from build123d import *

# Parameters (mm, degrees)
BASE_R                       = 9.5
BODY_DEPTH                   = 4.5
BASE_2_R                     = 4.53
SPLINE_EXTRUSION_BACK_DEPTH  = 1.34
BASE_3_R                     = 4.02
BASE_3_R_2                   = 3.27
SPLINE_EXTRUSION_FRONT_DEPTH = 0.6
FRONT_START                  = -0.9
FRONT_BASE_R                 = 3.27
FRONT_RECESSION_DEPTH        = 0.9
SPLINE_DEPTH                 = 4.3
CENTER_SCREW_HOLE_DEPTH      = 0.64
SCREW_HOLE_SKETCH_R          = 1
SCREW_HOLES_DEPTH            = 15.649423197


with BuildPart() as part:
    # base → body (new body)
    with BuildSketch(Plane.XY):
        Circle(BASE_R)
    extrude(amount=BODY_DEPTH)

    # base 2 → spline extrusion back (add)
    with BuildSketch(Plane(origin=(0, 0, 0), x_dir=(-1, 0, 0), z_dir=(0, 0, -1))):
        with Locations(Location((0, 0, 0), (0, 0, 180))):
            Circle(BASE_2_R)
    extrude(amount=SPLINE_EXTRUSION_BACK_DEPTH)

    # base 3 → spline extrusion front (add)
    with BuildSketch(Plane.XY.offset(4.5)):
        Circle(BASE_3_R)
        Circle(BASE_3_R_2, mode=Mode.SUBTRACT)
    extrude(amount=SPLINE_EXTRUSION_FRONT_DEPTH)

    # front base → front recession (cut)
    with BuildSketch(Plane.XY.offset(4.5).offset(FRONT_START)):
        Circle(FRONT_BASE_R)
    extrude(amount=FRONT_RECESSION_DEPTH, mode=Mode.SUBTRACT)

    # spline profile → spline (cut)
    with BuildSketch(Plane(origin=(0, 0, -1.34), x_dir=(-1, 0, 0), z_dir=(0, 0, -1))):
        Polygon((-0.325866407, 2.579498223), (0, 2.85), (0.325866407, 2.579498223), (0.708766178, 2.760462009), (0.957123837, 2.417418863), (1.372997971, 2.497474038), (1.528241656, 2.103444185), (1.950959252, 2.077560588), (2.003334431, 1.657302373), (2.406334588, 1.527106366), (2.352550336, 1.107026158), (2.710511071, 0.880698434), (2.553946852, 0.487191418), (2.844376176, 0.178952981), (2.594869494, -0.163255351), (2.799518665, -0.534036747), (2.472746942, -0.803444185), (2.5787571, -1.213470981), (2.195252606, -1.393149667), (2.195962742, -1.816658371), (1.779822475, -1.895318431), (1.675187969, -2.305698434), (1.252559553, -2.278397368), (1.049154975, -2.649862985), (0.646593707, -2.518316219), (0.357199716, -2.827526899), (0, -2.6), (-0.357199716, -2.827526899), (-0.646593707, -2.518316219), (-1.049154975, -2.649862985), (-1.252559553, -2.278397368), (-1.675187969, -2.305698434), (-1.779822475, -1.895318431), (-2.195962742, -1.816658371), (-2.195252606, -1.393149667), (-2.5787571, -1.213470981), (-2.472746942, -0.803444185), (-2.799518665, -0.534036747), (-2.594869494, -0.163255351), (-2.844376176, 0.178952981), (-2.553946852, 0.487191418), (-2.710511071, 0.880698434), (-2.352550336, 1.107026158), (-2.406334588, 1.527106366), (-2.003334431, 1.657302373), (-1.950959252, 2.077560588), (-1.528241656, 2.103444185), (-1.372997971, 2.497474038), (-0.957123837, 2.417418863), (-0.708766178, 2.760462009), align=None)
    extrude(amount=-SPLINE_DEPTH, mode=Mode.SUBTRACT)

    # center screw hole sketch → center screw hole (cut)
    with BuildSketch(Plane.XY.offset(3.6)):
        with BuildLine():
            Line((-0.55, -2.6), (0.55, -2.6))
            Line((0.55, -2.6), (0.55, -1.395528574))
            ThreePointArc((0.55, -1.395528574), (0, -1.5), (-0.55, -1.395528574))
            Line((-0.55, -1.395528574), (-0.55, -2.6))
        make_face()
        with BuildLine():
            ThreePointArc((-0.55, -1.395528574), (0, -1.5), (0.55, -1.395528574))
            ThreePointArc((0.55, -1.395528574), (1.239959677, -0.844097151), (1.5, 0))
            ThreePointArc((1.5, 0), (-0.844097151, 1.239959677), (-0.55, -1.395528574))
        make_face()
    extrude(amount=-CENTER_SCREW_HOLE_DEPTH, mode=Mode.SUBTRACT)

    # screw hole sketch → screw holes (cut, through all)
    with BuildSketch(Plane.XY.offset(4.5)):
        with Locations((0, 7)):
            Circle(SCREW_HOLE_SKETCH_R)
        with Locations((3.5, 6.062177826)):
            Circle(SCREW_HOLE_SKETCH_R)
        with Locations((6.062177826, 3.5)):
            Circle(SCREW_HOLE_SKETCH_R)
        with Locations((7, 0)):
            Circle(SCREW_HOLE_SKETCH_R)
        with Locations((6.062177826, -3.5)):
            Circle(SCREW_HOLE_SKETCH_R)
        with Locations((3.5, -6.062177826)):
            Circle(SCREW_HOLE_SKETCH_R)
        with Locations((0, -7)):
            Circle(SCREW_HOLE_SKETCH_R)
        with Locations((-3.5, -6.062177826)):
            Circle(SCREW_HOLE_SKETCH_R)
        with Locations((-6.062177826, -3.5)):
            Circle(SCREW_HOLE_SKETCH_R)
        with Locations((-7, 0)):
            Circle(SCREW_HOLE_SKETCH_R)
        with Locations((-6.062177826, 3.5)):
            Circle(SCREW_HOLE_SKETCH_R)
        with Locations((-3.5, 6.062177826)):
            Circle(SCREW_HOLE_SKETCH_R)
    extrude(amount=-SCREW_HOLES_DEPTH, mode=Mode.SUBTRACT)


solid = part.part
Geometry check sheet. Reference: the model listing, model coordinates, mm. A direction names the side the tool comes from. Give positions to 0.01 mm unless a question says otherwise; leave off trailing zeros. Loops run counter-clockwise (first coordinate to the right, second up) from the corner with the lowest first, then second, coordinate; pieces in that order, holes last. Notation, with made-up numbers: M 43.25,-27.75 L 50.25,-27.75 A22 ccw 50.25,-11.75 Z; hole C 80.25,1 d1. An arc over 180 degrees is marked long. Answer as a JSON object with one key per item and string values. Group by question number.
Item 1: Sectioned sample at B-B on z = 4. Give the number of separate pieces and of enclosed holes in the cut face, plus the area to 3 significant figures.
Item 2: Sectioned sample at D-D on x = 6.75. Record the boundary of the cut face in (y, z), plus the area to 3 significant figures.
Item 3: Mould release check, pull along Y, two halves, no side actions. Record for faces 1 (the cylindrical face through (4.38, -8.43, 2.22)), 2 (the cylindrical face through (-7.8, -0.6, 2.3)), 3 (the flat face through (-4.4, -2, 0)): pulls with the +Y half, pulls with the -Y half, needs draft (parallel to the pull), parting line crosses it, or undercut.
Item 4: Access from +Z, -Z, +X, -X, +Y, -Y to the whole of each face (thin tool, end or side, straight path). Record for faces 4 (the flat face through (1.2, 1.3, 2.96)), 5 (the cylindrical face through (3.283, 5.086, 2.282)), 6 (the flat face through (4, -2, 4.5)).
Item 5: Sectioned sample at C-C on x = -5.5. Record the boundary of the cut face in (y, z).
Item 6: Gauge pin test, flat ends, axial feed: pin 1 (1.8 mm diameter, centred on x = 3.5, y = 6.06, fed in from -Z); pin 2 (8.5 mm diameter, centred on x = 0, y = 0, fed in from -Z); pin 3 (2.5 mm diameter, centred on x = 0, y = 7, fed in from +Z); pin 4 (3 mm diameter, centred on y = 6, z = 0.5, fed in from -X). Record the tip position at first contact, or that the pin passes through.
Item 7: Sectioned sample at A-A on y = 3.5. Record the boundary of the cut face in (x, z), plus the area to 3 significant figures.
Item 8: Material ranges on L1, parallel to Y at x = -3.5, z = 1.2; L2, parallel to Y at x = 6.5, z = 1.75; L3, parallel to Z at x = 4.75, y = -7.5, recorded low to high.
Findings below:
{
 "1": {"separate pieces": "1", "enclosed holes": "13", "area": "212 mm2"},
 "2": {"outline": "M -6.68,0 L -4.23,0 L -4.23,4.5 L -6.68,4.5 Z; M -2.77,0 L -0.97,0 L -0.97,4.5 L -2.77,4.5 Z; M 0.97,0 L 2.77,0 L 2.77,4.5 L 0.97,4.5 Z; M 4.23,0 L 6.68,0 L 6.68,4.5 L 4.23,4.5 Z", "area": "38.4 mm2"},
 "3": {"face 1": "parting line crosses it", "face 2": "undercut", "face 3": "needs draft"},
 "4": {"face 4": "-Z", "face 5": "+Z, -Z", "face 6": "+Z"},
 "5": {"outline": "M -7.75,0 L -4.33,0 L -4.33,4.5 L -7.75,4.5 Z; M -2.67,0 L 2.67,0 L 2.67,4.5 L -2.67,4.5 Z; M 4.33,0 L 7.75,0 L 7.75,4.5 L 4.33,4.5 Z"},
 "6": {"pin 1": "through", "pin 2": "z = -1.34", "pin 3": "z = 4.5", "pin 4": "x = -8.37"},
 "7": {"outline": "M -8.83,0 L -7.06,0 L -7.06,4.5 L -8.83,4.5 Z; M -5.06,0 L -2.88,0 L -2.88,-1.34 L 2.88,-1.34 L 2.88,0 L 5.06,0 L 5.06,4.5 L 1.98,4.5 L 1.98,5.1 L -1.98,5.1 L -1.98,4.5 L -5.06,4.5 Z; M 7.06,0 L 8.83,0 L 8.83,4.5 L 7.06,4.5 Z", "area": "71.6 mm2"},
 "8": {"L1": "-8.83 to -7.06, -5.06 to 5.06, 7.06 to 8.83", "L2": "-6.93 to -4.4, -2.6 to -0.87, 0.87 to 2.6, 4.4 to 6.93", "L3": "0 to 4.5"}
}
